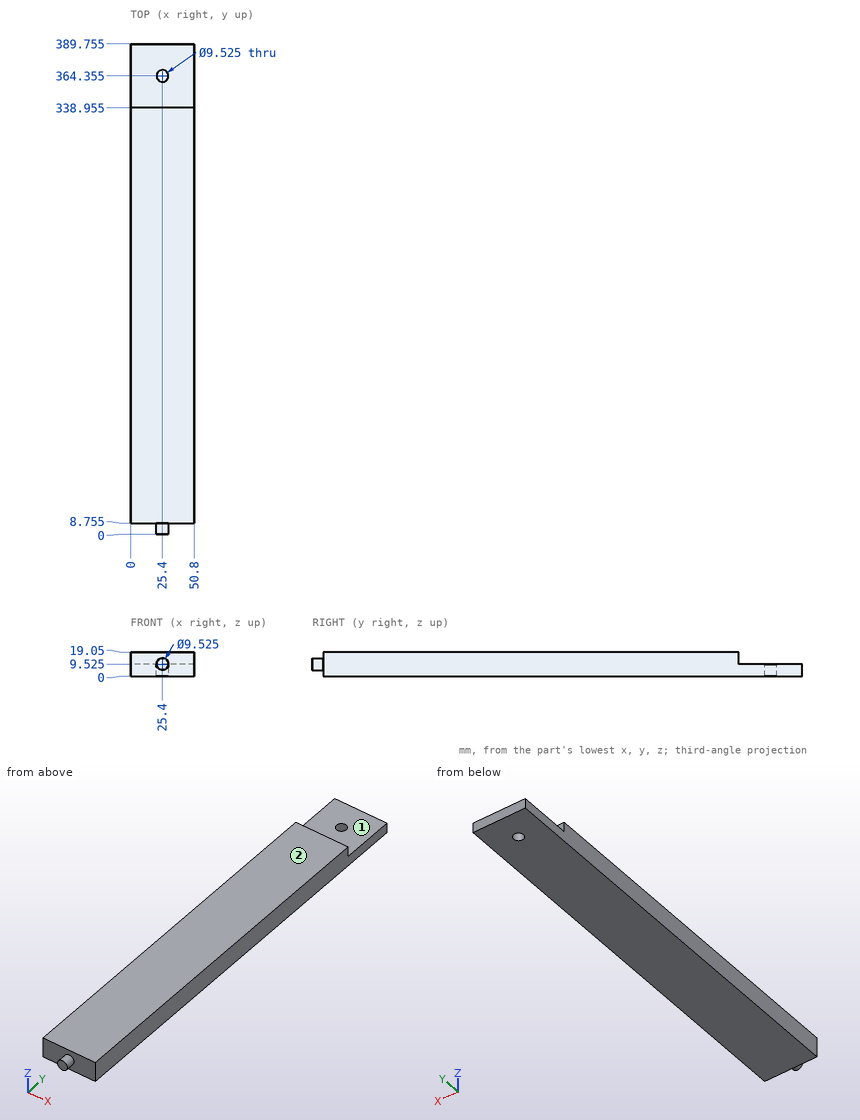
The figure shows three views and two pictorial views of one solid part (mm, origin at its lowest corner). Answer the questions. A direction names the side the tool comes from. Round coordinates to 2 decimals unless told otherwise and drop trailing zeros. Write item = value, one per line. Start each with the question number.
1) Straight lines are drawn through the part: L1, parallel to Y at x = 25.4, z = 2.25 (1 decimal); L2, parallel to Y at x = 25.4, z = 7 (1 decimal); L3, parallel to Y at x = 13.5, z = 17.5 (1 decimal). For each, find the intervals that lie inside material, in ascending order.
2) For the marked faces 1 and 2, determine the directions among +Z, -Z, +X, -X, +Y, -Y from which every point of the face is accessible in a straight line to the end or side of a thin tool.
3) Given pin 1 (5 mm diameter, centred on x = 32, y = 346, fed in from +Z) (3 decimals); pin 2 (5 mm diameter, centred on x = 15, z = 15, fed in from +Y) (1 decimal); pin 3 (5.5 mm diameter, centred on x = 38, z = 13, fed in from -Y) (1 decimal), each flat-ended and moving along its own axis, determine where each tip first touches the part or whether it passes through.
Results list:
q1.L1 = 8.8 to 359.6, 369.1 to 389.8
q1.L2 = 0 to 359.6, 369.1 to 389.8
q1.L3 = 8.8 to 339
q2.face_1 = +Z, +X, -X, +Y
q2.face_2 = +Z, +X, -X, +Y, -Y
q3.pin_1 = 9.525
q3.pin_2 = 339
q3.pin_3 = 8.8
